from build123d import *

# Parameters (mm, degrees)
F1_DEPTH = 34.925
F2_DEPTH = 2.0574
F3_DEPTH = 19.9898
F5_DEPTH = 25.4
F6_R     = 2.7432
F7_DEPTH = 6.35


with BuildPart() as f1:
    # F0 (on Top) → F1 (new body)
    with BuildSketch(Plane.XY):
        with BuildLine():
            ThreePointArc((-12.3453600693, -5.4627909314), (-13.1573816932, -3.0221361616), (-13.4917542774, -0.4717695609))
            ThreePointArc((-13.4917542774, -0.4717695609), (-13.6407310124, -0.1371936881), (-13.9803086533, 0))
            Line((-13.9803086533, 0), (-15.0031849319, 0))
            ThreePointArc((-15.0031849319, 0), (-15.3544396488, -0.1488568693), (-15.4917786026, -0.5047729485))
            ThreePointArc((-15.4917786026, -0.5047729485), (-4.6469501431, -14.7870164119), (12.418172291, -9.2757208319))
            ThreePointArc((12.418172291, -9.2757208319), (13.0538627177, -8.357431911), (13.6217786378, -7.395751939))
            ThreePointArc((13.6217786378, -7.395751939), (10.0950215904, 11.7618254999), (-9.3758099768, 12.3427787503))
            ThreePointArc((-9.3758099768, 12.3427787503), (-9.5654748501, 12.0117719837), (-9.4595485787, 11.645277961))
            Line((-9.4595485787, 11.645277961), (-8.8146223253, 10.8513346324))
            ThreePointArc((-8.8146223253, 10.8513346324), (-8.4940297415, 10.6742598531), (-8.140406046, 10.7695770301))
            ThreePointArc((-8.140406046, 10.7695770301), (-5.8949637992, 12.1449331742), (-3.4252504313, 13.0582410563))
            ThreePointArc((-3.4252504313, 13.0582410563), (12.1628613148, -5.8578839727), (-12.3453600693, -5.4627909314))
        make_face()
    extrude(amount=F1_DEPTH)

    # F0 (on Top) → F2 (join)
    with BuildSketch(Plane.XY):
        with BuildLine():
            Line((-10.812776349, -4.9974023539), (-12.3453600693, -5.4627909314))
            ThreePointArc((-12.3453600693, -5.4627909314), (12.1628613148, -5.8578839727), (-3.4252504313, 13.0582410563))
            Line((-3.4252504313, 13.0582410563), (-2.6983841205, 11.5607179889))
            ThreePointArc((-2.6983841205, 11.5607179889), (-2.4776784158, 11.3371662815), (-2.1665031819, 11.294080926))
            ThreePointArc((-2.1665031819, 11.294080926), (10.3351994601, -5.0431787713), (-10.2356285878, -5.2423188965))
            ThreePointArc((-10.2356285878, -5.2423188965), (-10.4797694006, -5.0151537509), (-10.812776349, -4.9974023539))
        make_face()
    extrude(amount=F2_DEPTH)

    # F0 (on Top) → F3 (join)
    with BuildSketch(Plane.XY):
        with BuildLine():
            ThreePointArc((13.6217786378, -7.395751939), (13.0538627177, -8.357431911), (12.418172291, -9.2757208319))
            Line((12.418172291, -9.2757208319), (34.5335465265, -23.8959513212))
            Line((34.5335465265, -23.8959513212), (35.7646481522, -22.033718493))
            Line((35.7646481522, -22.033718493), (13.6492739167, -7.4134880037))
            Line((13.6492739167, -7.4134880037), (13.6217786378, -7.395751939))
        make_face()
    extrude(amount=F3_DEPTH)

    # F4 (on face) → F5 (cut)
    with BuildSketch(Plane(origin=(-0.4904917501, -0.7419451164, 0), x_dir=(0.8341915273, -0.551474837, 0), z_dir=(-0.551474837, -0.8341915273, 0))):
        Polygon((41.9856077785, 5.0546), (36.6286821663, 0), (41.9856077785, 0), align=None)
        Polygon((41.9856077785, 19.9898), (36.6286821663, 19.9898), (41.9856077785, 14.9331064895), align=None)
    extrude(amount=-F5_DEPTH, mode=Mode.SUBTRACT)

    # F6 (on face) → F7 (cut)
    with BuildSketch(Plane(origin=(-0.4904917501, -0.7419451164, 0), x_dir=(0.8341915273, -0.551474837, 0), z_dir=(-0.551474837, -0.8341915273, 0))):
        with Locations((35.0006077785, 9.9949)):
            Circle(F6_R)
    extrude(amount=-F7_DEPTH, mode=Mode.SUBTRACT)


solid = f1.part
Source: CAD feature listing. Evaluate the final solid. Frame: model axes, mm. A direction names the side the tool comes from. Round coordinates to 2 decimals unless told otherwise and drop trailing zeros. Loops run counter-clockwise (first coordinate to the right, second up) from the corner with the lowest first, then second, coordinate; pieces in that order, holes last.
Q1. Access query for faces 4 (the face through (11, -4, 2.057)), 5 (the face through (23.321, -16.483, 9.855)), 6 (the face through (-3.067, 12.32, 1.014)). Directions: +Z, -Z, +X, -X, +Y, -Y. A direction counts if a zero-diameter tool reaches every point of the face in a straight line with its end or side. Return the directions, or none.
Q2. Mould query, pull axis X, two halves, no side actions, for faces 1 (the face through (10.487, -4.72, 1.014)), 2 (the face through (32.937, -21.521, 2.563)), 3 (the face through (22, -14, 19.99)). Classes: pulls with the +X half, pulls with the -X half, needs draft (parallel to the pull), parting line crosses it, or undercut.
Q3. Section C-C, the plane y = -10.5. Return loops of the section in (x, z) (3 decimals).
Q4. Ray query, line 1 (Y direction, x = 0, z = 1.3); line 2 (Y direction, x = 5.5, z = 5); line 3 (Z direction, x = 19, y = -12). Return the intervals inside material, ascending.
Q5. Section A-A, the plane x = 0. Return loops of the section in (y, z) (3 decimals), plus the area to 3 significant figures.
Q6. First-contact query: P1, Ø0.5, axis at x = -14.5, z = 17.5, coming from the +Y side; P2, Ø2, axis at x = 10.5, z = 30.5, coming from the +Y side; P3, Ø5, axis at y = -9.5, z = 21, coming from the -X side; P4, Ø21.5, axis at x = 0, y = 0, coming from the -Z side. Flat tips, straight axial feed; report the tip coordinate or a pass-through.
Solutions:
1. face 4: +Z
1. face 5: +Z, -Z, -Y
1. face 6: +Z, -Z
2. face 1: undercut
2. face 2: pulls with the +X half
2. face 3: needs draft
3. outline: (-11.402, 0) - (-4.69, 0) - (-4.69, 2.057) - (-8.485, 2.057) - (-8.485, 34.925) - (-11.402, 34.925) - close; (4.69, 0) - (11.402, 0) - (11.402, 34.925) - (8.485, 34.925) - (8.485, 2.057) - (4.69, 2.057) - close; (14.27, 0) - (18.318, 0) - (18.318, 19.99) - (14.27, 19.99) - close
4. line 1: y = -15.5 to -11.5, 11.5 to 15.5
4. line 2: y = -14.49 to -12.33, 12.33 to 14.49
4. line 3: z = 0 to 19.99
5. outline: (-15.5, 0) - (-11.5, 0) - (-11.5, 2.057) - (-13.5, 2.057) - (-13.5, 34.925) - (-15.5, 34.925) - close; (11.5, 0) - (15.5, 0) - (15.5, 34.925) - (13.5, 34.925) - (13.5, 2.057) - (11.5, 2.057) - close
5. area: 148 mm2
6. P1: stops at y = 0
6. P2: stops at y = 12.25
6. P3: stops at x = -13.83
6. P4: passes through
